from build123d import *

# Parameters (mm, degrees)
SKETCH_1_R          = 62.2
EXTRUDE_2_DEPTH     = 64
CUT_EXTRUDE_1_DEPTH = 122.437391276
FILLET_1_R          = 10
CHAMFER_1_SIZE      = 0.4


with BuildPart() as part:
    # 草图1 → 凸台-拉伸2 (new body)
    with BuildSketch(Plane(origin=(0, 0, 0), x_dir=(1, 0, 0), z_dir=(0, 1, 0))):
        with BuildLine():
            Line((-40, -51.488251087), (-40, -80))
            Line((-40, -80), (40, -80))
            Line((40, -80), (40, -51.488251087))
            ThreePointArc((40, -51.488251087), (0, 65.2), (-40, -51.488251087))
        make_face()
        with Locations(Location((0, 0, 0), (0, 0, 270))):
            Circle(SKETCH_1_R, mode=Mode.SUBTRACT)
    extrude(amount=EXTRUDE_2_DEPTH)

    # 草图2 → 切除-拉伸1 (cut, through all)
    with BuildSketch(Plane(origin=(0, 64, 0), x_dir=(1, 0, 0), z_dir=(0, 1, 0))):
        with BuildLine():
            Line((-30, -80), (30, -80))
            Line((30, -80), (30, -62.376598176))
            ThreePointArc((30, -62.376598176), (0, -69.215894128), (-30, -62.376598176))
            Line((-30, -62.376598176), (-30, -80))
        make_face()
    extrude(amount=-CUT_EXTRUDE_1_DEPTH, mode=Mode.SUBTRACT)

    # 圆角1
    fillet_1_edges = [part.edges().sort_by_distance(p)[0] for p in [
        (-30, 32, 62.376598176),
        (30, 32, 62.376598176),
        (-40, 32, 51.488251087),
        (40, 32, 51.488251087),
    ]]
    fillet(fillet_1_edges, radius=FILLET_1_R)

    # 倒角1
    chamfer_1_edges = [part.edges().sort_by_distance(p)[0] for p in [
        (0, 0, -62.2),
        (0, 64, -62.2),
        (-35, 64, 80),
        (35, 0, 80),
        (35, 64, 80),
        (-30, 32, 80),
        (30, 0, 78.324789245),
        (30, 32, 80),
        (30, 64, 78.324789245),
        (-30, 64, 78.324789245),
        (-30, 0, 78.324789245),
        (0, 64, 69.215894128),
        (0, 0, 69.215894128),
        (0, 0, -65.2),
        (0, 64, -65.2),
        (-40, 0, 68.084871372),
        (-40, 64, 68.084871372),
        (-26.113613559, 64, 68.736062883),
        (-26.113613559, 0, 68.736062883),
        (26.113613559, 64, 68.736062883),
        (26.113613559, 0, 68.736062883),
        (40.876147697, 0, 52.076416573),
        (40.876147697, 64, 52.076416573),
        (-40.876147697, 0, 52.076416573),
        (-40.876147697, 64, 52.076416573),
        (40, 64, 68.084871372),
        (-35, 0, 80),
        (40, 0, 68.084871372),
        (40, 32, 80),
        (-40, 32, 80),
    ]]
    chamfer(chamfer_1_edges, length=CHAMFER_1_SIZE)


solid = part.part
Geometry check sheet. Reference: the model listing, model coordinates, mm. A direction names the side the tool comes from. Round coordinates to 2 decimals unless told otherwise and drop trailing zeros. Loops run counter-clockwise (first coordinate to the right, second up) from the corner with the lowest first, then second, coordinate; pieces in that order, holes last.
Item 1: Thickness scan on line 1 (X direction, y = 40.5, z = 0); line 2 (X direction, y = 21.5, z = 2.5); line 3 (Z direction, x = 50, y = 41.5). Record the ranges inside material, lowest first.
Item 2: Cross-section at C-C on x = 0. Record the boundary of the cut face in (y, z), then the cut area to 3 significant figures.
Item 3: Gauge pin test, flat ends, axial feed: pin 1 (2 mm diameter, centred on y = 21, z = 2, fed in from -X); pin 2 (11.5 mm diameter, centred on y = 20.5, z = 72, fed in from +X); pin 3 (6 mm diameter, centred on x = -6.5, y = 11, fed in from -Z). Record the tip position at first contact, or that the pin passes through.
Item 4: Cross-section at B-B on y = 28. Record the boundary of the cut face in (x, z), then the cut area to 3 significant figures.
Item 5: Cross-section at A-A on z = 0. Record the boundary of the cut face in (x, y).
Item 6: Mould release check, pull along X, two halves, no side actions. Record for faces 1 (the cylindrical face through (2.203, 31.558, -65.163)), 2 (the cylindrical face through (-55.182, 31.558, 28.702)), 3 (the flat face through (35, 32, 80)): pulls with the +X half, pulls with the -X half, needs draft (parallel to the pull), parting line crosses it, or undercut.
Item 7: Access from +Z, -Z, +X, -X, +Y, -Y to the whole of each face (thin tool, end or side, straight path). Record for faces 4 (the flat face through (-20, 0, 61)), 5 (the flat face through (40, 32, 68)), 6 (the flat face through (-40, 32, 68)).
Answer sheet:
1. line 1: x = -65.2 to -62.2, 62.2 to 65.2
1. line 2: x = -65.15 to -62.15, 62.15 to 65.15
1. line 3: z = -41.85 to -37, 37 to 41.85
2. outline: (0, -64.8) - (0.4, -65.2) - (63.6, -65.2) - (64, -64.8) - (64, -62.6) - (63.6, -62.2) - (0.4, -62.2) - (0, -62.6) - close; (0, 62.6) - (0.4, 62.2) - (63.6, 62.2) - (64, 62.6) - (64, 68.82) - (63.6, 69.22) - (0.4, 69.22) - (0, 68.82) - close
2. area: 640 mm2
3. pin 1: stops at x = -65.19
3. pin 2: stops at x = 40
3. pin 3: stops at z = -65.11
4. outline: (-43.35, 48.7) arc R65.2 ccw (long way) to (43.35, 48.7) arc R10 cw to (40, 56.17) - (40, 79.6) - (39.6, 80) - (30.4, 80) - (30, 79.6) - (30, 76.65) arc R10 cw to (17.48, 66.97) arc R69.22 ccw to (-17.48, 66.97) arc R10 cw to (-30, 76.65) - (-30, 79.6) - (-30.4, 80) - (-39.6, 80) - (-40, 79.6) - (-40, 56.17) arc R10 cw to start; hole circle Ø124.4 at (0, 0)
4. area: 2,050 mm2
5. outline: (-65.2, 0.4) - (-64.8, 0) - (-62.6, 0) - (-62.2, 0.4) - (-62.2, 63.6) - (-62.6, 64) - (-64.8, 64) - (-65.2, 63.6) - close; (62.2, 0.4) - (62.6, 0) - (64.8, 0) - (65.2, 0.4) - (65.2, 63.6) - (64.8, 64) - (62.6, 64) - (62.2, 63.6) - close
6. face 1: parting line crosses it
6. face 2: undercut
6. face 3: needs draft
7. face 4: +Z, -Z, +X, -X, -Y
7. face 5: +Z, +X, +Y, -Y
7. face 6: +Z, -X, +Y, -Y
